Verification items for this drawing (mm, ordinates from the low corner). A direction names the side the tool comes from. Coordinates: 2 decimals unless noted, no trailing zeros. Loops run counter-clockwise (first coordinate to the right, second up) from the corner with the lowest first, then second, coordinate; pieces in that order, holes last. Notation, with made-up numbers: M -18.5,16.5 L 34.5,16.5 A22 cw 34.5,43.5 Z; hole C 73,63.5 d2. An arc over 180 degrees is marked long. Use CSV: the item, a comma, the result in double quotes.
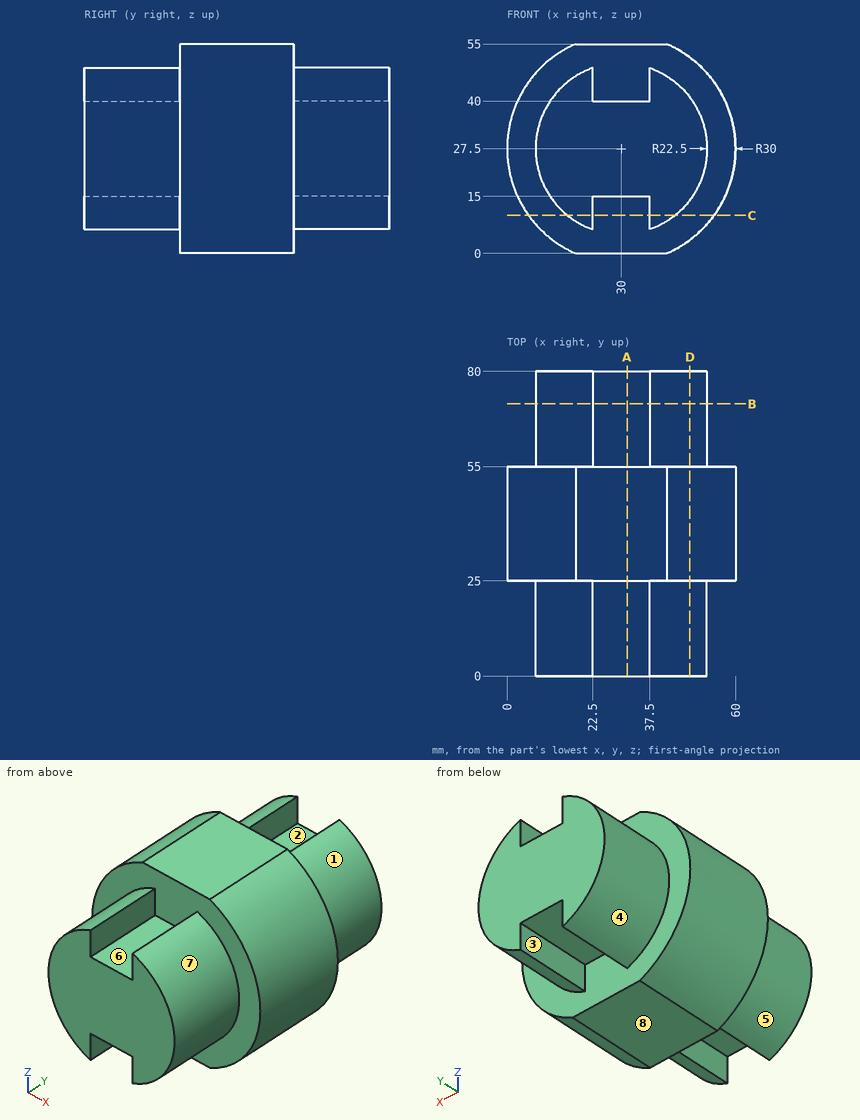
1. Set-up check for the marked faces 1, 2, 3, 4 and 5: record each of +Z, -Z, +X, -X, +Y, -Y from which the full face is reachable in a straight line by a thin tool's end or side.
The answers:
face 1,"+X, +Y"
face 2,"+Z, +Y"
face 3,"-Z, +Y"
face 4,"-X, +Y"
face 5,"-X, -Y"
2. Release check for a two-part mould opening along X. For the marked faces 6, 7 and 8 record: +X half, -X half, draft (parallel to the pull), parting line (faces both ways), or undercut.
The answers:
face 6,"undercut"
face 7,"+X half"
face 8,"draft"
3. Thickness scan on line 1 (Z direction, x = 28, y = 55.5); line 2 (X direction, y = 76, z = 13.5); line 3 (X direction, y = 77, z = 7). Record the ranges inside material, lowest first. Write a range as [from, to].
The answers:
line 1,"[15, 40]"
line 2,"[12.39, 22.5], [37.5, 47.61]"
line 3,"[20.73, 22.5], [37.5, 39.27]"
4. Section check D-D, the plane x = 48. Record the cut outline in (y, z), plus the area to 3 significant figures.
The answers:
outline,"M 0,14 L 25,14 L 25,3.5 L 55,3.5 L 55,14 L 80,14 L 80,41 L 55,41 L 55,51.5 L 25,51.5 L 25,41 L 0,41 Z"
area,"2,790 mm^2"
5. Section check A-A, the plane x = 31.5. Record the cut outline in (y, z), plus the area to 3 significant figures.
The answers:
outline,"M 0,15 L 25,15 L 25,0 L 55,0 L 55,15 L 80,15 L 80,40 L 55,40 L 55,55 L 25,55 L 25,40 L 0,40 Z"
area,"2,900 mm^2"
6. Section check B-B, the plane y = 71.5. Record the cut outline in (x, z).
The answers:
outline,"M 22.5,6.29 L 22.5,15 L 37.5,15 L 37.5,6.29 A22.5 ccw 37.5,48.71 L 37.5,40 L 22.5,40 L 22.5,48.71 A22.5 ccw Z"
7. Section check C-C, the plane z = 10. Record the cut outline in (x, y).
The answers:
outline,"M 5.63,25 L 15.86,25 L 15.86,0 L 22.5,0 L 22.5,25 L 37.5,25 L 37.5,0 L 44.14,0 L 44.14,25 L 54.37,25 L 54.37,55 L 44.14,55 L 44.14,80 L 37.5,80 L 37.5,55 L 22.5,55 L 22.5,80 L 15.86,80 L 15.86,55 L 5.63,55 Z"
8. Gauge pin test, flat ends, axial feed: P1, Ø4.5, axis at y = 66.5, z = 44.5, coming from the -X side; P2, Ø1.5, axis at x = 50, y = 39.5, coming from the +Z side; P3, Ø4.5, axis at x = 26.5, y = 16.5, coming from the -Z side. Record the tip position at first contact, or that the pin passes through.
The answers:
P1,"x = 13.01"
P2,"z = 50.51"
P3,"z = 15"
